Autodesk Inventor part; units mm, degrees
ref_plane "YZ Plane" through (0, 0, 0) normal (1, 0, 0) x (0, 1, 0)
ref_plane "XZ Plane" through (0, 0, 0) normal (0, 1, 0) x (-1, 0, 0)
ref_plane "XY Plane" through (0, 0, 0) normal (0, 0, 1) x (1, 0, 0)
sketch "Sketch1" plane through (0, 0, 0) normal (0, 0, 1) x (1, 0, 0)
  line L0 (-65, -20) -> (65, -20)
  line L1 (70, -15) -> (70, 15)
  line L2 (65, 20) -> (-65, 20)
  line L3 (-70, 15) -> (-70, -15)
  line L4 (65, 20) -> (65, 15)
  line L5 (65, 15) -> (70, 15)
  line L6 (0, 20) -> (0, -20)
  line L7 (65, -20) -> (65, -15)
  line L8 (65, -15) -> (70, -15)
  line L9 (-65, 20) -> (-65, 15)
  line L10 (-65, 15) -> (-70, 15)
  line L11 (-65, -20) -> (-65, -15)
  line L12 (-65, -15) -> (-70, -15)
  point P0 (0, 0)
extrude "Extrusion1" add sketch "Sketch1" along normal blind 4
sketch "Sketch2" plane through (0, 0, 0) normal (0, 0, -1) x (-1, 0, 0)
  arc A0 (-0.55, 20.0026) -> (0.55, 20.0026) centre (0, 19.05) ccw
  line L0 (-0.55, 21.2) -> (-5.25, 21.2)
  line L1 (5.25, 21.2) -> (0.55, 21.2)
  line L2 (6.1, 15.55) -> (6.1, 20.35)
  line L3 (0.55, -10.9) -> (5.25, -10.9)
  line L4 (-5.25, -10.9) -> (-0.55, -10.9)
  arc A1 (0.55, -9.7026) -> (-0.55, -9.7026) centre (0, -8.75) ccw
  line L5 (0.55, -10.9) -> (0.55, -9.7026)
  line L6 (-0.55, -9.7026) -> (-0.55, -10.9)
  line L7 (-6.1, -5.25) -> (-6.1, -10.05)
  line L8 (-6.1, 20.35) -> (-6.1, 15.55)
  arc A2 (-5.25, 21.2) -> (-6.1, 20.35) centre (-5.25, 20.35) ccw
  line L9 (-0.55, 21.2) -> (-0.55, 20.0026)
  line L10 (0.55, 20.0026) -> (0.55, 21.2)
  arc A3 (6.1, 20.35) -> (5.25, 21.2) centre (5.25, 20.35) ccw
  arc A4 (5.25, -10.9) -> (6.1, -10.05) centre (5.25, -10.05) ccw
  line L11 (6.1, -10.05) -> (6.1, -5.25)
  line L12 (6.1, -1.562) -> (6.1, -5.25)
  line L13 (6.1, 15.55) -> (6.1, 1.562)
  circle A5 centre (0, 0) radius 2.25
  line L14 (-6.1, -5.25) -> (-6.1, -1.562)
  line L15 (-6.1, 1.562) -> (-6.1, 15.55)
  line L16 (5.25, 16.4) -> (-5.25, 16.4)
  line L17 (-5.25, -6.1) -> (5.25, -6.1)
  arc A6 (5.25, -6.1) -> (6.1, -5.25) centre (5.25, -5.25) ccw
  arc A7 (-6.1, -5.25) -> (-5.25, -6.1) centre (-5.25, -5.25) ccw
  arc A8 (-6.1, -10.05) -> (-5.25, -10.9) centre (-5.25, -10.05) ccw
  arc A9 (6.1, 15.55) -> (5.25, 16.4) centre (5.25, 15.55) ccw
  arc A10 (-5.25, 16.4) -> (-6.1, 15.55) centre (-5.25, 15.55) ccw
  line L18 (-6.1, 1.562) -> (-6.1, -1.562)
  line L19 (6.1, 1.562) -> (6.1, -1.562)
  circle A11 centre (0, -8.75) radius 1.1
  circle A12 centre (0, 19.05) radius 1.1
  line L20 (-6.1, 15.55) -> (-6.1, 16.4)
  line L21 (-5.25, 16.4) -> (-6.1, 16.4)
  line L22 (5.25, 16.4) -> (6.1, 16.4)
  line L23 (6.1, 15.55) -> (6.1, 16.4)
  line L24 (5.25, -6.1) -> (6.1, -6.1)
  line L25 (-5.25, -6.1) -> (-6.1, -6.1)
  point P0 (-5.25, 21.2)
  point P1 (3.6026, 15)
  point P2 (3.95, 9.45)
  point P3 (0.55, 20.0026)
  point P4 (-0.55, -9.7026)
  point P5 (0.55, -9.7026)
sketch "Sketch3" plane through (0, 0, 0) normal (0, 0, -1) x (-1, 0, 0)
  line L0 (-65, 20) -> (65, 20)
  line L1 (-65, 20) -> (-20.7877, 20) construction
  line L2 (-20.7877, 20) -> (-20.7877, 27.1367) construction
  line L3 (-20.7877, 27.1367) -> (0, 27.1367) construction
  line L4 (0, 27.1367) -> (20.7877, 27.1367) construction
  line L5 (20.7877, 27.1367) -> (20.7877, 20) construction
  line L6 (20.7877, 20) -> (65, 20) construction
  spline S0 degree 4 poles (-65, 20) (-20.7877, 20) (-20.7877, 27.1367) (0, 27.1367) (20.7877, 27.1367) (20.7877, 20) (65, 20) knots 1 1 1 1 1 2 3 4 4 4 4 4
  line L7 (-65, 15) -> (-65, 20)
  line L8 (-65, 20) -> (65, 20)
  point P0 (0, 0)
extrude "Extrusion2" add sketch "Sketch3" against normal up to surface (4 mm away)
extrude "Extrusion3" cut sketch "Sketch2" against normal through all contours A12 A0 | L21 A10 L8 | A10 L16 A9 L13 L19 L12 A6 L17 A7 L14 L18 L15 | L2 A9 L22 | A7 L25 L7 | L11 L24 A6 | A1 A11 | A5
properties part number "sholder"
The model under review builds one solid part; all positions refer to its coordinate system, in mm. A direction names the side the tool comes from. Give positions to 0.01 mm unless a question says otherwise; leave off trailing zeros. Write each loop counter-clockwise with the first axis right and the second up, starting at its lowest first coordinate (ties: lowest second). Pieces come first, ordered by that corner, then holes.
1. Add section B-B, the plane z = 1.65. Count the separate pieces of the cut face and the enclosed holes in it, plus the area to 3 significant figures.
2. For P1, Ø1.5, axis at y = 18.5, z = 3, coming from the -X side; P2, Ø2, axis at x = 68.5, z = 2.5, coming from the -Y side; P3, Ø1.2, axis at y = -17, z = 2.5, coming from the +X side, all flat-tipped, find the tip position at first contact; note any pin that passes through.
3. Add section A-A, the plane y = 6. Write out the cut boundary in (x, z), plus the area to 3 significant figures.
4. Draft analysis for pull direction X (two halves, no side actions). For faces 4 (the flat face through (-65, -18, 2)), 5 (the flat face through (0, 16.4, 2)), 6 (the flat face through (65, 18, 2)), 7 (the flat face through (-6.1, 5, 2)), state which applies: +X half, -X half, draft (parallel to the pull), parting line (faces both ways), or undercut.
5. Tool access review of faces 1 (the flat face through (65, -18, 2)), 2 (the flat face through (0, -6.1, 2)), 3 (the flat face through (-65, 18, 2)): name each direction out of +Z, -Z, +X, -X, +Y, -Y from which nothing blocks a thin tool from reaching the whole face with its end or side.
6. Wall thickness on L1, parallel to Y at x = 0, z = 1.05; L2, parallel to X at y = 1, z = 3; L3, parallel to X at y = -8.5, z = 0.2: over which ranges is each line inside the solid? List them lowest first.
Worked answers:
1. separate pieces: 1
1. enclosed holes: 3
1. area: 5,540 mm2
2. P1: stops at x = -65
2. P2: stops at y = -15
2. P3: stops at x = 65
3. outline: (-70, 0) - (-6.1, 0) - (-6.1, 4) - (-70, 4) - close; (6.1, 0) - (70, 0) - (70, 4) - (6.1, 4) - close
3. area: 511 mm2
4. face 4: -X half
4. face 5: undercut
4. face 6: +X half
4. face 7: undercut
5. face 1: +Z, -Z, +X, -Y
5. face 2: +Z, -Z
5. face 3: +Z, -Z, -X, +Y
6. L1: y = -20 to -9.85, -7.65 to -6.1, 16.4 to 17.95, 20.15 to 27.03
6. L2: x = -70 to -6.1, 6.1 to 70
6. L3: x = -70 to -1.07, 1.07 to 70
